from build123d import *

# Parameters (mm, degrees)
SKETCH1_R           = 5.42927296
SKETCH1_R_2         = 5.999999996
SKETCH1_R_3         = 3
SKETCH1_R_4         = 18.05
BOSS_EXTRUDE1_DEPTH = 6.2


with BuildPart() as part:
    # Sketch1 → Boss-Extrude1 (new body)
    with BuildSketch(Plane.XY):
        with BuildLine():
            Line((39.614582687, 73.90348608), (39.884157083, 73.858752771))
            Line((39.884157083, 73.858752771), (70.59488962, 68.762598575))
            ThreePointArc((70.59488962, 68.762598575), (77.700603566, 64.224178317), (79.330264302, 55.951776308))
            Line((79.330264302, 55.951776308), (74.541718965, 33.423432184))
            Line((74.541718965, 33.423432184), (75.419376917, 32.916716129))
            ThreePointArc((75.419376917, 32.916716129), (79.892264849, 27.087535086), (78.933220793, 19.802872253))
            Line((78.933220793, 19.802872253), (68.367652451, 1.502771074))
            ThreePointArc((68.367652451, 1.502771074), (66.960524587, -6.114993434), (64.564182125, -13.481667564))
            Line((64.564182125, -13.481667564), (54.978164866, -55.003255407))
            Line((54.978164866, -55.003255407), (54.967848993, -84.703266118))
            Line((54.967848993, -84.703266118), (-77.032151007, -84.703266118))
            Line((-77.032151007, -84.703266118), (-77.032151007, -52.303266118))
            Line((-77.032151007, -52.303266118), (-77.032151007, -0.703266118))
            ThreePointArc((-77.032151007, -0.703266118), (-74.12202184, 7.271185396), (-67.432151007, 12.496733882))
            ThreePointArc((-67.432151007, 12.496733882), (-53.19307052, 29.559194605), (-60.354355055, 50.597136112))
            ThreePointArc((-60.354355055, 50.597136112), (-66.563388034, 74.831521387), (-43.015404957, 83.278415086))
            ThreePointArc((-43.015404957, 83.278415086), (-1.595924432, 79.511889283), (39.614582687, 73.90348608))
        make_face()
        with Locations(Location((68.504996686, 58.126398509, 0), (0, 0, 180))):
            Circle(SKETCH1_R, mode=Mode.SUBTRACT)
        with Locations(Location((-50.150905711, 66.123930347, 0), (0, 0, 180))):
            Circle(SKETCH1_R_2, mode=Mode.SUBTRACT)
        with Locations(Location((-6.283678939, 69.002872253, 0), (0, 0, 180))):
            Circle(SKETCH1_R_3, mode=Mode.SUBTRACT)
        with Locations(Location((26.219376917, -52.300183603, 0), (0, 0, 180))):
            Circle(SKETCH1_R_3, mode=Mode.SUBTRACT)
        with Locations(Location((70.619376917, 24.602872253, 0), (0, 0, 180))):
            Circle(SKETCH1_R_3, mode=Mode.SUBTRACT)
        with Locations(Location((-50.683678939, -7.900183603, 0), (0, 0, 180))):
            Circle(SKETCH1_R_3, mode=Mode.SUBTRACT)
        with Locations(Location((21.367848989, 28.096723532, 0), (0, 0, 180))):
            Circle(SKETCH1_R_4, mode=Mode.SUBTRACT)
        with BuildLine():
            ThreePointArc((-24.232151011, -59.303276516), (-18.438516483, -54.863340285), (-21.219337907, -48.114542837))
            Line((-21.219337907, -48.114542837), (-52.219337907, -30.114542837))
            ThreePointArc((-52.219337907, -30.114542837), (-58.225737603, -30.103426585), (-61.232151011, -35.303276516))
            Line((-61.232151011, -35.303276516), (-61.232151011, -53.303276516))
            ThreePointArc((-61.232151011, -53.303276516), (-59.474791698, -57.545917204), (-55.232151011, -59.303276516))
            Line((-55.232151011, -59.303276516), (-24.232151011, -59.303276516))
        make_face(mode=Mode.SUBTRACT)
    extrude(amount=BOSS_EXTRUDE1_DEPTH)


solid = part.part
Could you check a few things on this model? Use its own coordinates, in mm. A direction names the side the tool comes from. Coordinates: 2 decimals unless noted, no trailing zeros. Order: outer loops, then holes, each group sorted by start corner. A loop starts at its lowest first (then second) coordinate and runs counter-clockwise, first axis right, second up. Notation, with made-up numbers: (15, 34.25) - (28, 34.25) arc R5 cw to (28, 38.25) - close; hole circle Ø10 at (-36.5, 11.5). An arc over 180 degrees is marked (long way). Answer in a Markdown table with one row per item. Add a question column.
(1) Will these pins go through, and if not, where does the flat tip stop? pin 1 (3.5 mm diameter, centred on x = 70.62, y = 24.6, fed in from +Z); pin 2 (1.5 mm diameter, centred on y = 53.5, z = 1.5, fed in from -X); pin 3 (6 mm diameter, centred on x = -30.5, y = 24, fed in from -Z); pin 4 (3 mm diameter, centred on x = -46.5, z = 2.5, fed in from +Y).
(2) On a 3-axis mill with a long thin cutter (end or side, diameter ignored), from which of +Z, -Z, +X, -X, +Y, -Y can I reach the whole of each face in a straight line? I mean faces 1 (the face through (-61.232, -44, 3)), 2 (the face through (3, 1, 6.2)). Say none if no direction works.
(3) If we section it at B-B, the plane y = -44: Please give me the cut outline in (x, z).
(4) If we section it at C-C, the plane z = 3.75: State how many separate pieces and enclosed holes the cut face has, then the cut area to 3 significant figures.
(5) I need wall thicknesses on L1, parallel to X at y = 67.5, z = 1.25; L2, parallel to X at y = 27, z = 4; L3, parallel to Y at x = 21, z = 2.5. Which ranges of each line are inside material? Lowest first, please.
(6) If we section it at D-D, the plane x = -12.5: Please give me the cut outline in (y, z).
(7) If we mould it in two halves opening along Y, with no side actions, what happens to faces 3 (the face through (59.84, -33.95, 3.06)), 4 (the face through (-77.032, -43, 3)), 5 (the face through (72.831, 22.575, 3.057))? For each: released by +Y, released by -Y, zero draft, split by the parting line, or undercut.
(8) If we section it at A-A, the plane x = 31.5: Please give me the cut outline in (y, z), then the cut area to 3 significant figures.
Results are:
| question | item | result |
|---|---|---|
| 1 | pin 1 | passes through |
| 1 | pin 2 | stops at x = -64.44 |
| 1 | pin 3 | stops at z = 0 |
| 1 | pin 4 | stops at y = 84.58 |
| 2 | face 1 | +Z, -Z |
| 2 | face 2 | +Z, +X, -X, +Y, -Y |
| 3 | outline | (-77.03, 0) - (-61.23, 0) - (-61.23, 6.2) - (-77.03, 6.2) - close; (-28.31, 0) - (57.52, 0) - (57.52, 6.2) - (-28.31, 6.2) - close |
| 4 | separate pieces | 1 |
| 4 | enclosed holes | 8 |
| 4 | area | 20,100 mm2 |
| 5 | L1 | x = -68.68 to -55.99, -44.31 to -8.88, -3.69 to 74.15 |
| 5 | L2 | x = -53.82 to 3.35, 39.38 to 68.82, 72.42 to 79.92 |
| 5 | L3 | y = -84.7 to 10.05, 46.14 to 76.67 |
| 6 | outline | (-84.7, 0) - (80.68, 0) - (80.68, 6.2) - (-84.7, 6.2) - close |
| 7 | face 3 | released by -Y |
| 7 | face 4 | zero draft |
| 7 | face 5 | undercut |
| 8 | outline | (-84.7, 0) - (13.16, 0) - (13.16, 6.2) - (-84.7, 6.2) - close; (43.03, 0) - (75.16, 0) - (75.16, 6.2) - (43.03, 6.2) - close |
| 8 | area | 806 mm2 |
